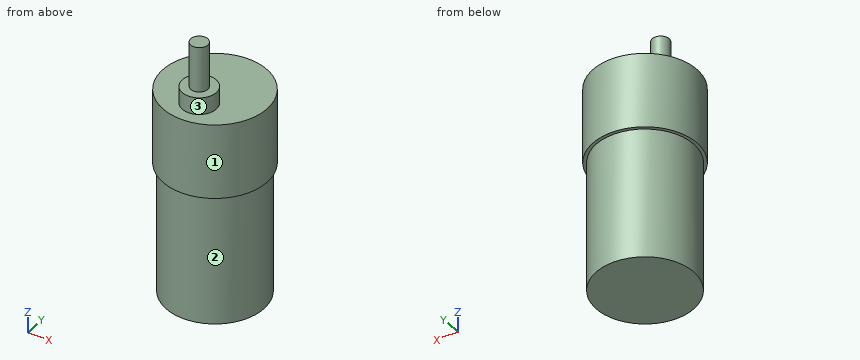
Autodesk Inventor part; units mm, degrees
ref_plane "YZ Plane" through (0, 0, 0) normal (1, 0, 0) x (0, 1, 0)
ref_plane "XZ Plane" through (0, 0, 0) normal (0, 1, 0) x (-1, 0, 0)
ref_plane "XY Plane" through (0, 0, 0) normal (0, 0, 1) x (1, 0, 0)
sketch "Sketch1" plane through (0, 0, 0) normal (0, 0, 1) x (1, 0, 0)
  circle A0 centre (0, 0) radius 18.4
  dimension "d0" = 36.8
extrude "Extrusion1" add sketch "Sketch1" along normal blind 26.5
sketch "Sketch2" plane through (0, 0, 0) normal (0, 0, -1) x (-1, 0, 0)
  circle A0 centre (0, 0) radius 17.25
  dimension "d3" = 34.5
extrude "Extrusion2" add sketch "Sketch2" along normal blind 46.1
sketch "Sketch5" plane through (0, 0, 26.5) normal (0, 0, 1) x (1, 0, 0)
  circle A0 centre (0, -8.4) radius 3
  circle A1 centre (0, -8.4) radius 6
  dimension "d7" = 6
  dimension "d8" = 12
extrude "Extrusion3" add sketch "Sketch5" along normal blind 6 contours A0 | A1
sketch "Sketch6" plane through (0, -8.4, 32.5) normal (0, 0, 1) x (1, 0, 0)
  circle A0 centre (0, 0) radius 3
  point P0 (0, 8.4)
  dimension "d11" = 6
extrude "Extrusion4" add sketch "Sketch6" along normal blind 16
properties part number "Big Motor"
Read the model definition and answer for the solid it produces. Units are mm, in the model's axes. Face numbers are marked on the shaded views. A direction names the side the tool comes from. Coordinates: 2 decimals unless noted, no trailing zeros. Write each loop counter-clockwise with the first axis right and the second up, starting at its lowest first coordinate (ties: lowest second). Pieces come first, ordered by that corner, then holes. Notation, with made-up numbers: M 68,55 L 87,55 A29 cw 87,80 Z; hole C 52.25,76.5 d5. An arc over 180 degrees is marked long. Use a Markdown table: item, result.
Q1. The part is cut by section C-C, the plane z = -6. Write down the section's boundary in (x, y), then the cut area to 3 significant figures.
Answer block:
| item | result |
|---|---|
| outline | C 0,0 d34.5 |
| area | 935 mm2 |
Q2. Which of the six approach directions +Z, -Z, +X, -X, +Y, -Y give full straight-line access (tool end or side, diameter ignored) to the marked faces 1, 2 and 3?
Answer block:
| item | result |
|---|---|
| face 1 | +Z, -Z |
| face 2 | -Z |
| face 3 | +Z |
Q3. Each of these flat-tipped pins is pushed along its axis until it touches: pin 1 Ø12 at (x, z) = (-9.5, 12.5) entering from -Y; pin 2 Ø3 at (y, z) = (7, -36.5) entering from -X; pin 3 Ø12 at (y, z) = (2.5, -18) entering from +X; pin 4 Ø3 at (y, z) = (0, 28.5) entering from -X. Where does it stop, or does it pass through?
Answer block:
| item | result |
|---|---|
| pin 1 | stops at y = -18.06 |
| pin 2 | stops at x = -16.35 |
| pin 3 | stops at x = 17.25 |
| pin 4 | passes through |
Q4. Straight lines are drawn through the part: L1, parallel to Y at x = 0.5, z = -28; L2, parallel to Z at x = -0.5, y = -3; L3, parallel to Z at x = 4, y = -3. For each, find the intervals that lie inside material, in ascending order. Write a range as [from, to].
Answer block:
| item | result |
|---|---|
| L1 | y = [-17.24, 17.24] |
| L2 | z = [-46.1, 32.5] |
| L3 | z = [-46.1, 26.5] |
Q5. The part is cut by section D-D, the plane y = -1. Write down the section's boundary in (x, z).
Answer block:
| item | result |
|---|---|
| outline | M -18.37,0 L -17.22,0 L -17.22,-46.1 L 17.22,-46.1 L 17.22,0 L 18.37,0 L 18.37,26.5 L -18.37,26.5 Z |
Q6. The part is cut by section A-A, the plane x = 0. Write down the section's boundary in (y, z).
Answer block:
| item | result |
|---|---|
| outline | M -18.4,0 L -17.25,0 L -17.25,-46.1 L 17.25,-46.1 L 17.25,0 L 18.4,0 L 18.4,26.5 L -2.4,26.5 L -2.4,32.5 L -5.4,32.5 L -5.4,48.5 L -11.4,48.5 L -11.4,32.5 L -14.4,32.5 L -14.4,26.5 L -18.4,26.5 Z |
Q7. The part is cut by section B-B, the plane y = -12.5. Write down the section's boundary in (x, z), then the cut area to 3 significant figures.
Answer block:
| item | result |
|---|---|
| outline | M -13.5,0 L -11.89,0 L -11.89,-46.1 L 11.89,-46.1 L 11.89,0 L 13.5,0 L 13.5,26.5 L 4.38,26.5 L 4.38,32.5 L -4.38,32.5 L -4.38,26.5 L -13.5,26.5 Z |
| area | 1,860 mm2 |
